For this review, use the dimensioned drawing (mm, ordinates from the lowest corner) and the shaded views. A direction names the side the tool comes from. Give positions to 0.01 mm unless a question says otherwise; leave off trailing zeros. Order: outer loops, then holes, each group sorted by start corner. A loop starts at its lowest first (then second) coordinate and runs counter-clockwise, first axis right, second up.
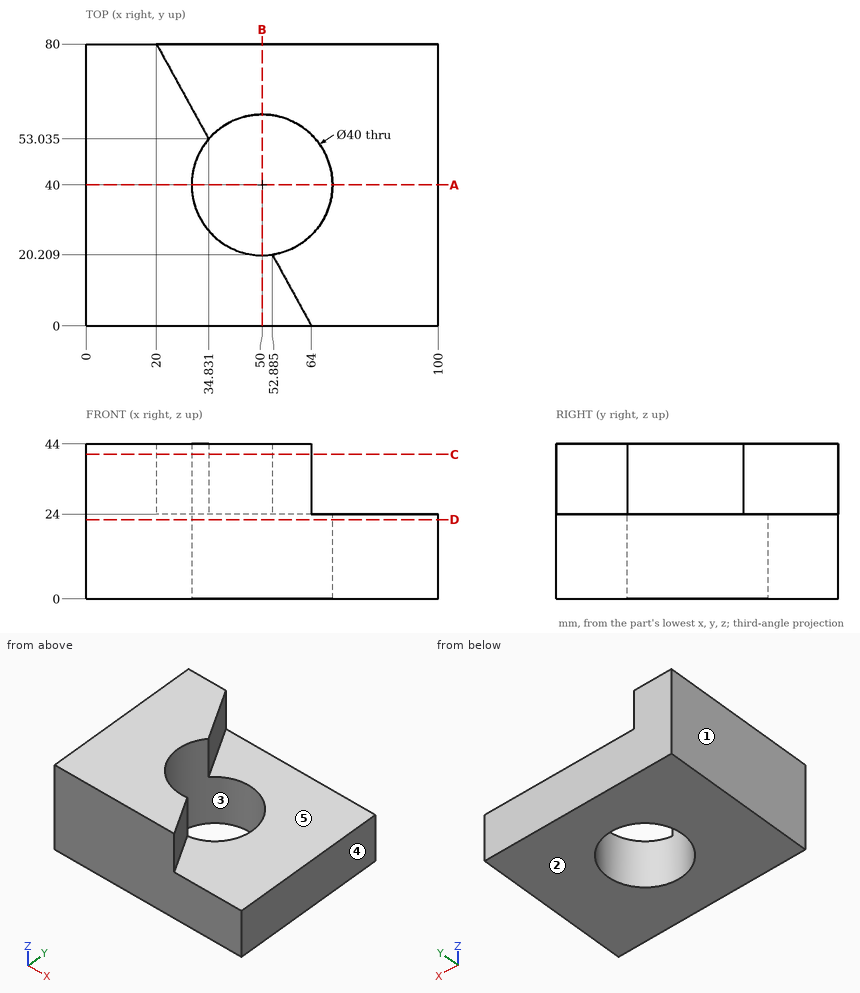
1. Draft analysis for pull direction X (two halves, no side actions). For the marked faces 1, 2 and 3, state which applies: pulls with the +X half, pulls with the -X half, needs draft (parallel to the pull), parting line crosses it, or undercut.
2. Take a section at A-A (y = 40). Write out the cut boundary in (x, z).
3. Take a section at B-B (x = 50). Write out the cut boundary in (y, z), and give its area (3 significant figures).
4. Take a section at C-C (z = 41). Write out the cut boundary in (x, y) (1 decimal).
5. Insertion check: pin 1 (6 mm diameter, centred on x = 71.5, y = 48, fed in from +Z). The pin has a flat end and moves straight along its axis. Give the tip position at first contact, or say it passes through.
6. Take a section at D-D (z = 22.5). Write out the cut boundary in (x, y), and give its area (3 significant figures).
7. To check wall thickness, follow line 1 (Y direction, x = 50, z = 12.5); line 2 (X direction, y = 40, z = 18); line 3 (Z direction, x = 81.5, y = 36.5). State the ranges of each line that lie inside material, in increasing order.
8. For the marked faces 4 and 5, list the 3-axis set-ups (+Z, -Z, +X, -X, +Y, -Y) from which the entire face can be reached by the end or side of a thin tool; tool diameter is ignored.
Answer:
1. face 1: pulls with the -X half
1. face 2: needs draft
1. face 3: undercut
2. outline: (0, 0) - (30, 0) - (30, 44) - (0, 44) - close; (70, 0) - (100, 0) - (100, 24) - (70, 24) - close
3. outline: (0, 0) - (20, 0) - (20, 44) - (0, 44) - close; (60, 0) - (80, 0) - (80, 24) - (60, 24) - close
3. area: 1,360 mm2
4. outline: (0, 0) - (64, 0) - (52.9, 20.2) arc R20 cw to (34.8, 53) - (20, 80) - (0, 80) - close
5. pin 1: stops at z = 24
6. outline: (0, 0) - (100, 0) - (100, 80) - (0, 80) - close; hole circle Ø40 at (50, 40)
6. area: 6,740 mm2
7. line 1: y = 0 to 20, 60 to 80
7. line 2: x = 0 to 30, 70 to 100
7. line 3: z = 0 to 24
8. face 4: +Z, -Z, +X, +Y, -Y
8. face 5: +Z, +X, +Y
